The drawing under review shows one solid part. Ordinate dimensions are in mm from its lowest x, y, z. Give positions to 0.01 mm unless a question says otherwise; leave off trailing zeros. Order: outer loops, then holes, each group sorted by start corner. A loop starts at its lowest first (then second) coordinate and runs counter-clockwise, first axis right, second up. Notation, with made-up numbers: (25, -30) - (62, -30) arc R18 ccw to (62, -10) - close; hole circle Ø2 at (41, 65). An arc over 180 degrees is marked (long way). Use CSV: the item, a comma, the result in double quotes.
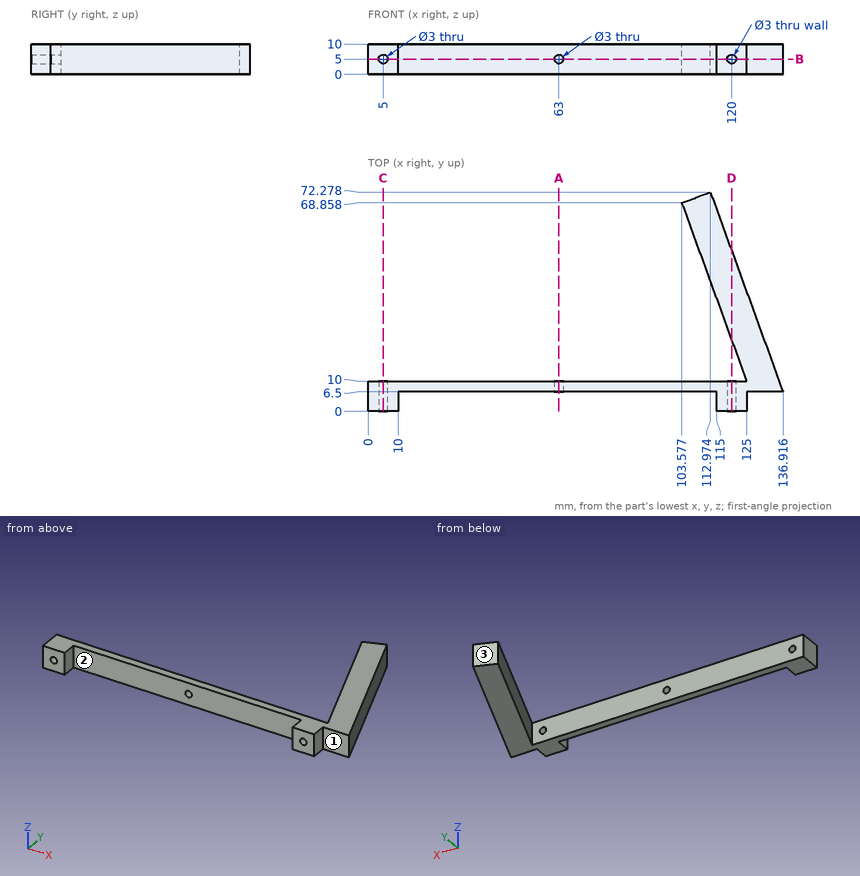
Item 1: Take a section at D-D, the plane x = 120. Give the boundary of the cut face in (y, z) (1 decimal).
Results list:
outline,"(0, 0) - (10, 0) - (10, 3.5) - (0, 3.5) - close; (0, 6.5) - (10, 6.5) - (10, 10) - (0, 10) - close; (23.7, 0) - (53, 0) - (53, 10) - (23.7, 10) - close"
Item 2: Take a section at C-C, the plane x = 5. Give the boundary of the cut face in (y, z).
Results list:
outline,"(0, 0) - (10, 0) - (10, 3.5) - (0, 3.5) - close; (0, 6.5) - (10, 6.5) - (10, 10) - (0, 10) - close"
Item 3: Wall thickness on L1, parallel to Z at x = 5, y = 4.75; L2, parallel to X at y = 9, z = 4.75 (1 decimal); L3, parallel to Y at x = 29.5, z = 3.75: over which ranges is each line inside the solid? List them lowest first.
Results list:
L1,"z = 0 to 3.5, 6.5 to 10"
L2,"x = 0 to 3.5, 6.5 to 61.5, 64.5 to 118.5, 121.5 to 136"
L3,"y = 6.5 to 10"
Item 4: Take a section at B-B, the plane z = 5. Give the boundary of the cut face in (x, y) (1 decimal), and give its area (3 significant figures).
Results list:
outline,"(0, 0) - (3.5, 0) - (3.5, 10) - (0, 10) - close; (6.5, 0) - (10, 0) - (10, 6.5) - (61.5, 6.5) - (61.5, 10) - (6.5, 10) - close; (64.5, 6.5) - (115, 6.5) - (115, 0) - (118.5, 0) - (118.5, 10) - (64.5, 10) - close; (103.6, 68.9) - (125, 10) - (121.5, 10) - (121.5, 0) - (125, 0) - (125, 6.5) - (136.9, 6.5) - (113, 72.3) - close"
area,"1,180 mm2"
Item 5: Take a section at A-A, the plane x = 63. Give the boundary of the cut face in (y, z), and give its area (3 significant figures).
Results list:
outline,"(6.5, 0) - (10, 0) - (10, 3.5) - (6.5, 3.5) - close; (6.5, 6.5) - (10, 6.5) - (10, 10) - (6.5, 10) - close"
area,"24.5 mm2"
Item 6: Mouldability with a two-part tool opening along X and no side actions: class the marked faces 1, 2 and 3 as pulls with the +X half, pulls with the -X half, needs draft (parallel to the pull), parting line crosses it, or undercut.
Results list:
face 1,"needs draft"
face 2,"undercut"
face 3,"pulls with the -X half"
Item 7: Clearance check with flat-ended pins moving along their axes: pin 1 (4 mm diameter, centred on y = 44.5, z = 3, fed in from +X); pin 2 (4 mm diameter, centred on x = 89.5, z = 7.5, fed in from -Y); pin 3 (2.5 mm diameter, centred on x = 5, z = 5, fed in from -Y) (3 decimals); pin 4 (5 mm diameter, centred on y = 36, z = 3.5, fed in from +X). State where each tip first meets the part, or that it passes through.
Results list:
pin 1,"stops at x = 123.81"
pin 2,"stops at y = 6.5"
pin 3,"passes through"
pin 4,"stops at x = 127.09"
